Source: CAD feature listing. Evaluate the final solid. Frame: model axes, mm. A direction names the side the tool comes from. Coordinates: 2 decimals unless noted, no trailing zeros. Loops run counter-clockwise (first coordinate to the right, second up) from the corner with the lowest first, then second, coordinate; pieces in that order, holes last.
Item 1: Line query: probe 1 along Y at (x, z) = (27, 1); probe 2 along X at (y, z) = (4.75, 0.75); probe 3 along Z at (x, y) = (35.5, 2.5). Output: solid intervals per line, ascending.
Item 2: Reachability of faces 5 (the flat face through (18.8, 1.6, 1.1)), 6 (the flat face through (6, 5, 1)), 7 (the flat face through (45.58, 3.02, 1.06)) from +Z, -Z, +X, -X, +Y, -Y: full face, straight path, thin tool, end or side. Return the list, or none.
Item 3: Section query C-C, the plane x = 36. Return the cut outline in (y, z).
Item 4: Pull-direction query (X, two-part tool) for faces 1 (the flat face through (45.6, 4.7, 1.1)), 2 (the cylindrical face through (25.5, 3.9, 1.1)), 3 (the flat face through (6, 0, 1)), 4 (the flat face through (40, 4, 3)); classes: +X half, -X half, draft (parallel to the pull), parting line (faces both ways), or undercut.
Item 5: Section query B-B, the plane z = -0.5. Return the cut outline in (x, y), then the cut area to 3 significant figures.
Item 6: Pin query (flat end, axial travel): pin 1 Ø0.6 at (y, z) = (5, -1) entering from -X; pin 2 Ø1.5 at (y, z) = (5.5, 2) entering from +X; pin 3 Ø2.5 at (x, z) = (6, 1) entering from -Y; pin 4 Ø2.5 at (x, y) = (28, 3) entering from -Z. Return the tip coordinate at first contact, or that it passes through.
Item 7: Section query A-A, the plane x = 30. Return the cut outline in (y, z), then the cut area to 3 significant figures.
```python
from build123d import *

# Parameters (mm, degrees)
F0_W      = 40
F0_H      = 7.8
F1_DEPTH  = 2.2
F2_W      = 7.8
F2_H      = 6.2
F3_DEPTH  = 6
F5_DEPTH  = 25
F7_DEPTH  = 25
F8_R      = 1
F10_DEPTH = 25
F12_DEPTH = 25


with BuildPart() as f1:
    # F0 (on Top) → F1 (new body)
    with BuildSketch(Plane.XY):
        with Locations((20, 3.9)):
            Rectangle(F0_W, F0_H)
    extrude(amount=F1_DEPTH)

    # F2 (on face) → F3 (join)
    with BuildSketch(Plane.YZ.offset(40)):
        with Locations((3.9, 1.1)):
            Rectangle(F2_W, F2_H)
    extrude(amount=F3_DEPTH)

    # F4 (on face) → F5 (cut)
    with BuildSketch(Plane(origin=(0, 0, -2), x_dir=(1, 0, 0), z_dir=(0, 0, -1))):
        Polygon((46, -1.829873), (46, 0), (45.176316, -0.90971), align=None)
        Polygon((46, -7.8), (46, -6.802324), (45.176316, -7.8), align=None)
        Polygon((46, -6.802324), (46, -5.144841), (45.176316, -5.882161), align=None)
        Polygon((46, -5.144841), (46, -3.487357), (45.176316, -4.224677), align=None)
        Polygon((46, -3.487357), (46, -1.829873), (45.176316, -2.567193), align=None)
    extrude(amount=-F5_DEPTH, mode=Mode.SUBTRACT)

    # F6 (on face) → F7 (cut)
    with BuildSketch(Plane(origin=(0, 0, 0), x_dir=(1, 0, 0), z_dir=(0, 0, -1))):
        Polygon((12, 0), (15, -3.5), (22, 0), align=None)
    extrude(amount=-F7_DEPTH, mode=Mode.SUBTRACT)

    # F8
    f8_edges = [f1.edges().sort_by_distance(p)[0] for p in [
        (15, 3.5, 1.1),
    ]]
    fillet(f8_edges, radius=F8_R)

    # F9 (on face) → F10 (cut)
    with BuildSketch(Plane(origin=(0, 0, 0), x_dir=(1, 0, 0), z_dir=(0, 0, -1))):
        with BuildLine():
            Line((8.4, -2.8), (2.9, -2.8))
            ThreePointArc((2.9, -2.8), (1.8, -3.9), (2.9, -5))
            Line((2.9, -5), (8.4, -5))
            ThreePointArc((8.4, -5), (9.5, -3.9), (8.4, -2.8))
        make_face()
    extrude(amount=-F10_DEPTH, mode=Mode.SUBTRACT)

    # F11 (on face) → F12 (cut)
    with BuildSketch(Plane(origin=(0, 0, 0), x_dir=(1, 0, 0), z_dir=(0, 0, -1))):
        with BuildLine():
            Line((32.1, -2.8), (26.6, -2.8))
            ThreePointArc((26.6, -2.8), (25.5, -3.9), (26.6, -5))
            Line((26.6, -5), (32.1, -5))
            ThreePointArc((32.1, -5), (33.2, -3.9), (32.1, -2.8))
        make_face()
    extrude(amount=-F12_DEPTH, mode=Mode.SUBTRACT)


solid = f1.part
```
Verdict:
1. probe 1: y = 0 to 2.8, 5 to 7.8
1. probe 2: x = 0 to 2.2, 9.1 to 25.9, 32.8 to 45.65
1. probe 3: z = 0 to 2.2
2. face 5: +Z, -Z, -Y
2. face 6: +Z, -Z
2. face 7: +Z, -Z, +X
3. outline: (0, 0) - (7.8, 0) - (7.8, 2.2) - (0, 2.2) - close
4. face 1: +X half
4. face 2: undercut
4. face 3: draft
4. face 4: -X half
5. outline: (40, 0) - (46, 0) - (45.18, 0.91) - (46, 1.83) - (45.18, 2.57) - (46, 3.49) - (45.18, 4.22) - (46, 5.14) - (45.18, 5.88) - (46, 6.8) - (45.18, 7.8) - (40, 7.8) - close
5. area: 43.6 mm2
6. pin 1: stops at x = 40
6. pin 2: stops at x = 46
6. pin 3: stops at y = 0
6. pin 4: stops at z = 0
7. outline: (0, 0) - (2.8, 0) - (2.8, 2.2) - (0, 2.2) - close; (5, 0) - (7.8, 0) - (7.8, 2.2) - (5, 2.2) - close
7. area: 12.3 mm2
